Read the model definition and answer for the solid it produces. Units are mm, in the model's axes. A direction names the side the tool comes from. Coordinates: 2 decimals unless noted, no trailing zeros. Order: outer loops, then holes, each group sorted by start corner. A loop starts at its lowest first (then second) coordinate and runs counter-clockwise, first axis right, second up.
```python
from build123d import *

# Parameters (mm, degrees)
SKETCH2_R           = 30
SKETCH2_R_2         = 25
SKETCH2_W           = 48.360210917
SKETCH2_H           = 12.7
SKETCH2_R_3         = 3.175
SKETCH2_W_2         = 3.81
SKETCH2_H_2         = 5.08
BOSS_EXTRUDE1_DEPTH = 11
SKETCH2_3_W         = 3.81
SKETCH2_3_H         = 5.08
CUT_EXTRUDE1_DEPTH  = 10


with BuildPart() as part:
    # Sketch2 → Boss-Extrude1 (new body)
    # profile 1 of 9: a face of its own
    with BuildSketch(Plane.XY):
        with Locations((-124.832414552, 99.62481555)):
            Circle(SKETCH2_R)
        with Locations((-124.832414552, 99.62481555)):
            Circle(SKETCH2_R_2, mode=Mode.SUBTRACT)
    # profile 2 of 9: a face of its own
    with BuildSketch(Plane.XY):
        with Locations((-124.832414553, 99.62481555)):
            Rectangle(SKETCH2_W, SKETCH2_H)
        with Locations((-124.832414552, 99.62481555)):
            Circle(SKETCH2_R_3, mode=Mode.SUBTRACT)
    # profile 3 of 9: a face of its own
    with BuildSketch(Plane.XY):
        with BuildLine():
            Line((-149.012520011, 93.27481555), (-149.012520011, 105.97481555))
            ThreePointArc((-149.012520011, 105.97481555), (-149.832414552, 99.62481555), (-149.012520011, 93.27481555))
        make_face()
    # profile 4 of 9: a face of its own
    with BuildSketch(Plane.XY):
        with BuildLine():
            ThreePointArc((-99.832414552, 99.62481555), (-100.038235432, 102.826171788), (-100.652309094, 105.97481555))
            Line((-100.652309094, 105.97481555), (-100.652309094, 93.27481555))
            ThreePointArc((-100.652309094, 93.27481555), (-100.038235432, 96.423459312), (-99.832414552, 99.62481555))
        make_face()
    # profile 5 of 9: a face of its own
    with BuildSketch(Plane.XY):
        with BuildLine():
            Line((-126.737414552, 97.08481555), (-126.737414552, 102.16481555))
            ThreePointArc((-126.737414552, 102.16481555), (-128.007414552, 99.62481555), (-126.737414552, 97.08481555))
        make_face()
    # profile 6 of 9: a face of its own
    with BuildSketch(Plane.XY):
        with BuildLine():
            ThreePointArc((-121.657414552, 99.62481555), (-121.992608221, 101.044718716), (-122.927414552, 102.16481555))
            Line((-122.927414552, 102.16481555), (-122.927414552, 97.08481555))
            ThreePointArc((-122.927414552, 97.08481555), (-121.992608221, 98.204912384), (-121.657414552, 99.62481555))
        make_face()
    # profile 7 of 9: a face of its own
    with BuildSketch(Plane.XY):
        with BuildLine():
            ThreePointArc((-122.927414552, 102.16481555), (-124.832414552, 102.79981555), (-126.737414552, 102.16481555))
            Line((-126.737414552, 102.16481555), (-122.927414552, 102.16481555))
        make_face()
    # profile 8 of 9: a face of its own
    with BuildSketch(Plane.XY):
        with Locations((-124.832414552, 99.62481555)):
            Rectangle(SKETCH2_W_2, SKETCH2_H_2)
    # profile 9 of 9: a face of its own
    with BuildSketch(Plane.XY):
        with BuildLine():
            Line((-122.927414552, 97.08481555), (-126.737414552, 97.08481555))
            ThreePointArc((-126.737414552, 97.08481555), (-124.832414552, 96.44981555), (-122.927414552, 97.08481555))
        make_face()
    extrude(amount=-BOSS_EXTRUDE1_DEPTH)

    # Sketch2_3 → Cut-Extrude1 (cut)
    with BuildSketch(Plane.XY):
        with Locations((-124.832414552, 99.62481555)):
            Rectangle(SKETCH2_3_W, SKETCH2_3_H)
        with BuildLine():
            Line((-122.927414552, 97.08481555), (-126.737414552, 97.08481555))
            ThreePointArc((-126.737414552, 97.08481555), (-124.832414552, 96.44981555), (-122.927414552, 97.08481555))
        make_face()
        with BuildLine():
            ThreePointArc((-122.927414552, 102.16481555), (-124.832414552, 102.79981555), (-126.737414552, 102.16481555))
            Line((-126.737414552, 102.16481555), (-122.927414552, 102.16481555))
        make_face()
    extrude(amount=-CUT_EXTRUDE1_DEPTH, mode=Mode.SUBTRACT)


solid = part.part
```
1) A cutting plane is placed at A-A, the plane y = 88. Determine the outline of the cut face in (x, z), and give its area (3 significant figures).
A:
outline: (-152.49, -11) - (-146.97, -11) - (-146.97, 0) - (-152.49, 0) - close; (-102.7, -11) - (-97.18, -11) - (-97.18, 0) - (-102.7, 0) - close
area: 122 mm2
2) A cutting plane is placed at D-D, the plane y = 110.5. Determine the outline of the cut face in (x, z), and give its area (3 significant figures).
A:
outline: (-152.79, -11) - (-147.34, -11) - (-147.34, 0) - (-152.79, 0) - close; (-102.32, -11) - (-96.87, -11) - (-96.87, 0) - (-102.32, 0) - close
area: 120 mm2
3) A cutting plane is placed at B-B, the plane x = -144. Determine the outline of the cut face in (y, z).
A:
outline: (76.55, -11) - (83.57, -11) - (83.57, 0) - (76.55, 0) - close; (93.27, -11) - (105.97, -11) - (105.97, 0) - (93.27, 0) - close; (115.67, -11) - (122.7, -11) - (122.7, 0) - (115.67, 0) - close
4) A cutting plane is placed at C-C, the plane z = -4.25. Determine the outline of the cut face in (x, y) (3 decimals), and give its area (3 significant figures).
A:
outline: circle Ø60 at (-124.832, 99.625); hole (-149.013, 93.275) arc R25 ccw to (-100.652, 93.275) - close; hole (-149.013, 105.975) - (-100.652, 105.975) arc R25 ccw to start; hole (-126.737, 97.085) arc R3.175 ccw to (-122.927, 97.085) - (-122.927, 102.165) arc R3.175 ccw to (-126.737, 102.165) - close
area: 1,470 mm2
5) Which of the six approach directions +Z, -Z, +X, -X, +Y, -Y give full straight-line access (tool end or side, diameter ignored) to faces 1 (the flat face through (-119, 100, 0)), 2 (the flat face through (-125, 93.275, -5)), 3 (the cylindrical face through (-124.8, 102.8, -4.9))?
A:
face 1: +Z, +X, -X, +Y, -Y
face 2: +Z, -Z
face 3: +Z
6) Flat-ended cylindrical pins translate along their axes: pin 1 Ø4 at (x, z) = (-146, -4) entering from -Y; pin 2 Ø5.5 at (x, z) = (-115, -5) entering from -Y; pin 3 Ø1.5 at (y, z) = (104, -7.5) entering from -X. Find the tip coordinate at first contact, or state that the pin passes through.
A:
pin 1: stops at y = 76.55
pin 2: stops at y = 70.47
pin 3: stops at x = -154.61
7) Determine the mould class of faces 4 (the flat face through (-125, 105.975, -5)), 5 (the cylindrical face through (-154.803, 100.944, -5.423)), 6 (the cylindrical face through (-124.86, 96.45, -4.93)), 7 (the flat face through (-125, 100, -11)) for opening direction Y: pulls with the +Y half, pulls with the -Y half, needs draft (parallel to the pull), parting line crosses it, or undercut.
A:
face 4: undercut
face 5: parting line crosses it
face 6: undercut
face 7: needs draft
8) Straight lines are drawn through the part: line 1 (Y direction, x = -103.5, z = -9.25); line 2 (Y direction, x = -138, z = -2); line 3 (X direction, y = 100, z = -7). For each, find the intervals that lie inside material, in ascending order.
A:
line 1: y = 78.53 to 86.59, 93.27 to 105.97, 112.66 to 120.72
line 2: y = 72.67 to 78.37, 93.27 to 105.97, 120.88 to 126.58
line 3: x = -154.83 to -126.74, -122.93 to -94.83
